from build123d import *

# Parameters (mm, degrees)
BOSS_EXTRUDE1_DEPTH = 25
FILLET1_R           = 5


with BuildPart() as part:
    # Sketch1 → Boss-Extrude1 (new body)
    with BuildSketch(Plane(origin=(0, 0, 0), x_dir=(1, 0, 0), z_dir=(0, 1, 0))):
        with BuildLine():
            Line((-34.8, 0), (-34.8, -23.97))
            Line((-34.8, -23.97), (-32.158644924, -23.97))
            ThreePointArc((-32.158644924, -23.97), (-30.548804634, -23.156766295), (-30.248140727, -21.378414239))
            ThreePointArc((-30.248140727, -21.378414239), (-17.4, -3.95), (-4.551859273, -21.378414239))
            ThreePointArc((-4.551859273, -21.378414239), (-4.251195366, -23.156766295), (-2.641355076, -23.97))
            Line((-2.641355076, -23.97), (0, -23.97))
            Line((0, -23.97), (0, 0))
            Line((0, 0), (-34.8, 0))
        make_face()
    extrude(amount=BOSS_EXTRUDE1_DEPTH)

    # Fillet1
    fillet1_edges = [part.edges().sort_by_distance(p)[0] for p in [
        (0, 12.5, 0),
        (-34.8, 12.5, 0),
    ]]
    fillet(fillet1_edges, radius=FILLET1_R)


solid = part.part
Input: part model. Units: mm. Frame: model coordinates. A direction names the side the tool comes from. Coordinates: 2 decimals unless noted, no trailing zeros. Order: outer loops, then holes, each group sorted by start corner. A loop starts at its lowest first (then second) coordinate and runs counter-clockwise, first axis right, second up.
1. Contact query for flat-ended pins moving along their axis: P1, Ø6, axis at x = -28.5, y = 3.5, coming from the +Z side; P2, Ø4, axis at x = -15, y = 4.5, coming from the +Z side. Output: stop coordinate, or through.
Checked values:
P1: stops at z = 23.86
P2: stops at z = 4.69
2. Cut plane B-B, the plane y = 7.5. Return loops of the section in (x, z).
Checked values:
outline: (-34.8, 5) arc R5 ccw to (-29.8, 0) - (-5, 0) arc R5 ccw to (0, 5) - (0, 23.97) - (-2.64, 23.97) arc R2 ccw to (-4.55, 21.38) arc R13.45 cw (long way) to (-30.25, 21.38) arc R2 ccw to (-32.16, 23.97) - (-34.8, 23.97) - close
3. Ray query, line 1 along X through (y, z) = (18.25, 17.4); line 2 along Z through (x, y) = (-17.4, 12.25); line 3 along X through (y, z) = (12.75, 7.75). Return the intervals inside material, ascending.
Checked values:
line 1: x = -34.8 to -30.85, -3.95 to 0
line 2: z = 0 to 3.95
line 3: x = -34.8 to -26.77, -8.03 to 0
4. Cut plane D-D, the plane z = 3.25. Return loops of the section in (x, y).
Checked values:
outline: (-34.48, 0) - (-0.32, 0) - (-0.32, 25) - (-34.48, 25) - close
5. Access query for faces 1 (the flat face through (-33, 12, 23.97)), 2 (the cylindrical face through (-4.267, 12.325, 23.136)). Directions: +Z, -Z, +X, -X, +Y, -Y. A direction counts if a zero-diameter tool reaches every point of the face in a straight line with its end or side. Return the directions, or none.
Checked values:
face 1: +Z, +X, -X, +Y, -Y
face 2: +Y, -Y
6. Cut plane C-C, the plane x = -17.4. Return loops of the section in (y, z), plus the area to 4 significant figures.
Checked values:
outline: (0, 0) - (25, 0) - (25, 3.95) - (0, 3.95) - close
area: 98.75 mm2
7. Draft query along X for faces 3 (the cylindrical face through (-33.37, 12.68, 1.5)), 4 (the cylindrical face through (-17.752, 12.325, 3.955)), 5 (the flat face through (-17.6, 25, 3.8)). Return one class per face: +X half, -X half, draft (parallel to the pull), parting line (faces both ways), or undercut.
Checked values:
face 3: -X half
face 4: undercut
face 5: draft
8. Cut plane A-A, the plane z = 17.4. Return loops of the section in (x, y), plus the area to 4 significant figures.
Checked values:
outline: (-34.8, 0) - (-30.85, 0) - (-30.85, 25) - (-34.8, 25) - close; (-3.95, 0) - (0, 0) - (0, 25) - (-3.95, 25) - close
area: 197.5 mm2
